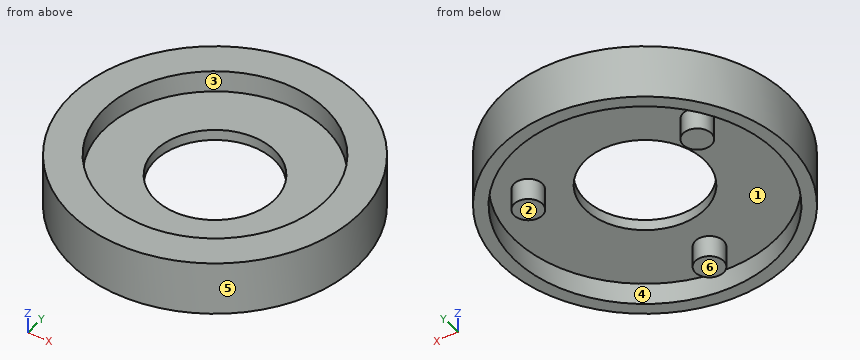
```python
from build123d import *

# Parameters (mm, degrees)
SKETCH_R        = 13.25
PAD_DEPTH       = 5
SKETCH001_R     = 10.2
POCKET_DEPTH    = 2
SKETCH002_R     = 12.05
POCKET001_DEPTH = 2
SKETCH003_R     = 5.5
POCKET002_DEPTH = 5
SKETCH004_R     = 1.3
PAD001_DEPTH    = 2


with BuildPart() as part:
    # Sketch → Pad (new body)
    with BuildSketch(Plane.XY):
        Circle(SKETCH_R)
    extrude(amount=PAD_DEPTH)

    # Sketch001 → Pocket (cut)
    with BuildSketch(Plane.XY.offset(5)):
        Circle(SKETCH001_R)
    extrude(amount=-POCKET_DEPTH, mode=Mode.SUBTRACT)

    # Sketch002 → Pocket001 (cut)
    with BuildSketch(Plane(origin=(0, 0, 0), x_dir=(1, 0, 0), z_dir=(0, 0, -1))):
        Circle(SKETCH002_R)
    extrude(amount=-POCKET001_DEPTH, mode=Mode.SUBTRACT)

    # Sketch003 → Pocket002 (cut)
    with BuildSketch(Plane(origin=(0, 0, 2), x_dir=(1, 0, 0), z_dir=(0, 0, -1))):
        Circle(SKETCH003_R)
    extrude(amount=-POCKET002_DEPTH, mode=Mode.SUBTRACT)

    # Sketch004 → Pad001 (new body)
    with BuildSketch(Plane(origin=(0, 0, 2), x_dir=(1, 0, 0), z_dir=(0, 0, -1))):
        with Locations((0, 9.00666)):
            Circle(SKETCH004_R)
        with Locations((7.8, -4.50333)):
            Circle(SKETCH004_R)
        with Locations((-7.8, -4.50333)):
            Circle(SKETCH004_R)
    extrude(amount=PAD001_DEPTH)


solid = part.part
```
Check sheet for the modelled part. Datum: model origin and axes. Units: mm. Face numbers are marked on the shaded views. A direction names the side the tool comes from. Round coordinates to 2 decimals unless told otherwise and drop trailing zeros. Loops run counter-clockwise (first coordinate to the right, second up) from the corner with the lowest first, then second, coordinate; pieces in that order, holes last. Notation, with made-up numbers: (-25, 7) - (-4, 7) arc R13 ccw to (-4, 17) - close; hole circle Ø4 at (-1, 28). An arc over 180 degrees is marked (long way). Write item = value, one per line. Start each with the question number.
Q1. Section check B-B (x = 0). Record the boundary of the cut face in (y, z).
Q2. Thickness scan on L1, parallel to Y at x = 0, z = 4.5; L2, parallel to Z at x = 10.25, y = 2.25; L3, parallel to Z at x = -3, y = -8.25. Record the ranges inside material, lowest first.
Q3. Access from +Z, -Z, +X, -X, +Y, -Y to the whole of each face (thin tool, end or side, straight path). Record for the marked faces 1, 2 and 3.
Q4. Depth check by flat-ended pin: P1, Ø14.5, axis at x = 0, y = 0, coming from the -Z side; P2, Ø10, axis at x = 0.5, y = 1, coming from the +Z side; P3, Ø1.5, axis at y = 8, z = 1, coming from the +X side. Enter the tip coordinate at first touch or a pass-through.
Q5. Section check A-A (y = 0). Record the boundary of the cut face in (x, z).
Q6. Section check C-C (z = 0.4). Record the boundary of the cut face in (x, y), plus the area to 3 significant figures.
Q7. Section check D-D (z = 4.1). Record the boundary of the cut face in (x, y), plus the area to 3 significant figures.
Q8. Release check for a two-part mould opening along X. For the marked faces 4, 5 and 6 record: pulls with the +X half, pulls with the -X half, needs draft (parallel to the pull), parting line crosses it, or undercut.
Derived:
q1.outline = (-13.25, 0) - (-12.05, 0) - (-12.05, 2) - (-10.31, 2) - (-10.31, 0) - (-7.71, 0) - (-7.71, 2) - (-5.5, 2) - (-5.5, 3) - (-10.2, 3) - (-10.2, 5) - (-13.25, 5) - close; (5.5, 2) - (12.05, 2) - (12.05, 0) - (13.25, 0) - (13.25, 5) - (10.2, 5) - (10.2, 3) - (5.5, 3) - close
q2.L1 = -13.25 to -10.2, 10.2 to 13.25
q2.L2 = 2 to 5
q2.L3 = 2 to 3
q3.face_1 = -Z
q3.face_2 = -Z, +X, -X, +Y, -Y
q3.face_3 = +Z
q4.P1 = 2
q4.P2 = 3
q4.P3 = 11.09
q5.outline = (-13.25, 0) - (-12.05, 0) - (-12.05, 2) - (-5.5, 2) - (-5.5, 3) - (-10.2, 3) - (-10.2, 5) - (-13.25, 5) - close; (5.5, 2) - (12.05, 2) - (12.05, 0) - (13.25, 0) - (13.25, 5) - (10.2, 5) - (10.2, 3) - (5.5, 3) - close
q6.outline = circle Ø26.5 at (0, 0); circle Ø2.6 at (-7.8, 4.5); circle Ø2.6 at (0, -9.01); circle Ø2.6 at (7.8, 4.5); hole circle Ø24.1 at (0, 0)
q6.area = 111 mm^2
q7.outline = circle Ø26.5 at (0, 0); hole circle Ø20.4 at (0, 0)
q7.area = 225 mm^2
q8.face_4 = undercut
q8.face_5 = parting line crosses it
q8.face_6 = needs draft
